from build123d import *

# Parameters (mm, degrees)
EXTRUDE_1_DEPTH     = 1.2
SKETCH_2_R          = 1.375
CUT_EXTRUDE_1_DEPTH = 1.2
SKETCH_3_W          = 6
SKETCH_3_H          = 13
EXTRUDE_2_DEPTH     = 5
SKETCH_4_W          = 6
SKETCH_4_H          = 5
EXTRUDE_3_DEPTH     = 0.3
SKETCH_5_W          = 8
SKETCH_5_H          = 7
EXTRUDE_4_DEPTH     = 5.5
SKETCH_6_W          = 12
SKETCH_6_H          = 8.2
EXTRUDE_5_DEPTH     = 5.1
SKETCH_7_W          = 12
SKETCH_7_H          = 8.2
EXTRUDE_6_DEPTH     = 5.1
SKETCH_8_W          = 5.7
SKETCH_8_H          = 7.6
EXTRUDE_7_DEPTH     = 2.4
SKETCH_9_W          = 7.6
SKETCH_9_H          = 2.4
EXTRUDE_8_DEPTH     = 0.7
SKETCH_10_W         = 12
SKETCH_10_H         = 5.1
SKETCH_10_W_2       = 8
SKETCH_10_H_2       = 5.5
CUT_EXTRUDE_2_DEPTH = 0.5
SKETCH_11_W         = 51.4
SKETCH_11_H         = 5.1
EXTRUDE_9_DEPTH     = 8.5
SKETCH_12_W         = 6.2
SKETCH_12_H         = 6.2
EXTRUDE_10_DEPTH    = 3.5
SKETCH_13_R         = 1.75
EXTRUDE_11_DEPTH    = 1.5
SKETCH_14_W         = 2
SKETCH_14_H         = 2
EXTRUDE_12_DEPTH    = 1
SKETCH_15_R         = 2.75
SKETCH_15_R_2       = 1.55
EXTRUDE_13_DEPTH    = 2


with BuildPart() as part:
    # 草图1 → 凸台-拉伸1 (new body)
    with BuildSketch(Plane(origin=(0, 0, 0), x_dir=(1, 0, 0), z_dir=(0, 1, 0))):
        with BuildLine():
            Line((-29.5, 15), (29.5, 15))
            ThreePointArc((29.5, 15), (31.621320344, 14.121320344), (32.5, 12))
            Line((32.5, 12), (32.5, -12))
            ThreePointArc((32.5, -12), (31.621320344, -14.121320344), (29.5, -15))
            Line((29.5, -15), (-29.5, -15))
            ThreePointArc((-29.5, -15), (-31.621320344, -14.121320344), (-32.5, -12))
            Line((-32.5, -12), (-32.5, 12))
            ThreePointArc((-32.5, 12), (-31.621320344, 14.121320344), (-29.5, 15))
        make_face()
    extrude(amount=EXTRUDE_1_DEPTH)

    # 草图2 → 切除-拉伸1 (cut)
    with BuildSketch(Plane(origin=(0, 1.2, 0), x_dir=(1, 0, 0), z_dir=(0, 1, 0))):
        with Locations(Location((29, -11.5, 0), (0, 0, 270))):
            Circle(SKETCH_2_R)
        with Locations(Location((29, 11.5, 0), (0, 0, 270))):
            Circle(SKETCH_2_R)
        with Locations(Location((-29, -11.5, 0), (0, 0, 270))):
            Circle(SKETCH_2_R)
        with Locations(Location((-29, 11.5, 0), (0, 0, 270))):
            Circle(SKETCH_2_R)
    extrude(amount=-CUT_EXTRUDE_1_DEPTH, mode=Mode.SUBTRACT)

    # 草图3 → 凸台-拉伸2 (add)
    with BuildSketch(Plane(origin=(0, 1.2, 0), x_dir=(1, 0, 0), z_dir=(0, 1, 0))):
        with Locations((22.3, -8.5)):
            Rectangle(SKETCH_3_W, SKETCH_3_H)
    extrude(amount=EXTRUDE_2_DEPTH)

    # 草图4 → 凸台-拉伸3 (add)
    with BuildSketch(Plane.XY.offset(15)):
        with Locations((22.3, 3.7)):
            Rectangle(SKETCH_4_W, SKETCH_4_H)
    extrude(amount=EXTRUDE_3_DEPTH)

    # 草图5 → 凸台-拉伸4 (add)
    with BuildSketch(Plane(origin=(0, 1.2, 0), x_dir=(1, 0, 0), z_dir=(0, 1, 0))):
        with Locations((5.6, -11.5)):
            Rectangle(SKETCH_5_W, SKETCH_5_H)
    extrude(amount=EXTRUDE_4_DEPTH)

    # 草图6 → 凸台-拉伸5 (add)
    with BuildSketch(Plane(origin=(0, 1.2, 0), x_dir=(1, 0, 0), z_dir=(0, 1, 0))):
        with Locations((-5.9, -10.9)):
            Rectangle(SKETCH_6_W, SKETCH_6_H)
    extrude(amount=EXTRUDE_5_DEPTH)

    # 草图7 → 凸台-拉伸6 (add)
    with BuildSketch(Plane(origin=(0, 1.2, 0), x_dir=(1, 0, 0), z_dir=(0, 1, 0))):
        with Locations((-19.45, -10.9)):
            Rectangle(SKETCH_7_W, SKETCH_7_H)
    extrude(amount=EXTRUDE_6_DEPTH)

    # 草图8 → 凸台-拉伸7 (add)
    with BuildSketch(Plane(origin=(0, 1.2, 0), x_dir=(1, 0, 0), z_dir=(0, 1, 0))):
        with Locations((-29.65, -1.5)):
            Rectangle(SKETCH_8_W, SKETCH_8_H)
    extrude(amount=EXTRUDE_7_DEPTH)

    # 草图9 → 凸台-拉伸8 (add)
    with BuildSketch(Plane.ZY.offset(32.5)):
        with Locations((1.5, 2.4)):
            Rectangle(SKETCH_9_W, SKETCH_9_H)
    extrude(amount=EXTRUDE_8_DEPTH)

    # 草图10 → 切除-拉伸2 (cut)
    with BuildSketch(Plane.XY.offset(15)):
        with Locations((-19.45, 3.75)):
            Rectangle(SKETCH_10_W, SKETCH_10_H)
        with Locations((-5.9, 3.75)):
            Rectangle(SKETCH_10_W, SKETCH_10_H)
        with Locations((5.6, 3.95)):
            Rectangle(SKETCH_10_W_2, SKETCH_10_H_2)
    extrude(amount=-CUT_EXTRUDE_2_DEPTH, mode=Mode.SUBTRACT)

    # 草图11 → 凸台-拉伸9 (add)
    with BuildSketch(Plane.XZ):
        with Locations((-0.05, -11.55)):
            Rectangle(SKETCH_11_W, SKETCH_11_H)
    extrude(amount=EXTRUDE_9_DEPTH)

    # 草图12 → 凸台-拉伸10 (add)
    with BuildSketch(Plane(origin=(0, 1.2, 0), x_dir=(1, 0, 0), z_dir=(0, 1, 0))):
        with Locations((-16.2, 2.6)):
            Rectangle(SKETCH_12_W, SKETCH_12_H)
    extrude(amount=EXTRUDE_10_DEPTH)

    # 草图13 → 凸台-拉伸11 (add)
    with BuildSketch(Plane(origin=(0, 4.7, 0), x_dir=(1, 0, 0), z_dir=(0, 1, 0))):
        with Locations(Location((-16.2, 2.6, 0), (0, 0, 270))):
            Circle(SKETCH_13_R)
    extrude(amount=EXTRUDE_11_DEPTH)

    # 草图14 → 凸台-拉伸12 (add)
    with BuildSketch(Plane(origin=(0, 1.2, 0), x_dir=(1, 0, 0), z_dir=(0, 1, 0))):
        with Locations((3.2, 3.22)):
            Rectangle(SKETCH_14_W, SKETCH_14_H)
        with Locations((0, 3.22)):
            Rectangle(SKETCH_14_W, SKETCH_14_H)
        with Locations((-3.2, 3.22)):
            Rectangle(SKETCH_14_W, SKETCH_14_H)
    extrude(amount=EXTRUDE_12_DEPTH)

    # 草图15 → 凸台-拉伸13 (add)
    with BuildSketch(Plane.XY.offset(15.3)):
        with Locations(Location((22.3, 3.7, 0), (0, 0, 114.619977329))):
            Circle(SKETCH_15_R)
        with Locations((22.3, 3.7)):
            Circle(SKETCH_15_R_2, mode=Mode.SUBTRACT)
    extrude(amount=EXTRUDE_13_DEPTH)


solid = part.part
The listing builds one solid part. Answer for the finished solid, in the listing's coordinates (mm). A direction names the side the tool comes from. Round coordinates to 2 decimals unless told otherwise and drop trailing zeros. Order: outer loops, then holes, each group sorted by start corner. A loop starts at its lowest first (then second) coordinate and runs counter-clockwise, first axis right, second up. Notation, with made-up numbers: (-2.75, 51.25) -> (21.25, 51.25) arc R17 ccw to (21.25, 60.25) -> close; hole circle Ø3 at (-11.75, -7). An arc over 180 degrees is marked (long way). Put each result on its own line as item: value.
Q1. Each of these flat-tipped pins is pushed along its axis until it touches: P1, Ø9, axis at x = 4.5, z = -1.5, coming from the +Y side; P2, Ø12, axis at x = -16.5, z = 7.5, coming from the -Y side; P3, Ø1.9, axis at x = -15, z = -2, coming from the +Y side; P4, Ø1, axis at y = -1, z = -7.5, coming from the -X side. Where does it stop, or does it pass through?
Results list:
P1: y = 2.2
P2: y = 0
P3: y = 6.2
P4: through
Q2. Which of the six approach directions +Z, -Z, +X, -X, +Y, -Y give full straight-line access (tool end or side, diameter ignored) to faces 1 (the flat face through (-19.3, 3, -3)), 2 (the flat face through (-16, 6.2, -3)), 3 (the flat face through (19.3, 4, 9))?
Results list:
face 1: -Z, +Y
face 2: -Z, +X, -X, +Y
face 3: +Z, -Z, +Y
Q3. Section D-D, the plane y = -1 is taken. Write down the section's boundary in (x, z), and give its area (3 significant figures).
Results list:
outline: (-25.75, -14.1) -> (25.65, -14.1) -> (25.65, -9) -> (-25.75, -9) -> close
area: 262 mm^2
Q4. Consider line 1 along X through (y, z) = (0.7, -11.5) (3 decimals); line 2 along X through (y, z) = (4.5, 12.5); line 3 along X through (y, z) = (1.25, -1). Determine where each line is inside the solid, lowest interval first.
Results list:
line 1: -32.5 to -30.375, -27.625 to 27.625, 30.375 to 32.5
line 2: -25.45 to -13.45, -11.9 to 0.1, 1.6 to 9.6, 19.3 to 25.3
line 3: -33.2 to -26.8, -19.3 to -13.1
Q5. Determine the mould class of faces 4 (the flat face through (-6, 4, 14.5)), 5 (the flat face through (-16, 3, -5.7)), 6 (the flat face through (-25.75, -4, -12)), 7 (the flat face through (-20, 4, 6.8)) for opening direction Z: pulls with the +Z half, pulls with the -Z half, needs draft (parallel to the pull), parting line crosses it, or undercut.
Results list:
face 4: pulls with the +Z half
face 5: pulls with the -Z half
face 6: needs draft
face 7: undercut
Q6. Section C-C, the plane y = 3 is taken. Count the separate pieces of the cut face and the enclosed holes in it, and give its area (3 significant figures).
Results list:
separate pieces: 6
enclosed holes: 0
area: 409 mm^2
Q7. Section A-A, the plane z = -11 is taken. Write down the section's boundary in (x, y).
Results list:
outline: (-32.5, 0) -> (-30.28, 0) -> (-30.28, 1.2) -> (-32.5, 1.2) -> close; (-27.72, 0) -> (-25.75, 0) -> (-25.75, -8.5) -> (25.65, -8.5) -> (25.65, 0) -> (27.72, 0) -> (27.72, 1.2) -> (-27.72, 1.2) -> close; (30.28, 0) -> (32.5, 0) -> (32.5, 1.2) -> (30.28, 1.2) -> close
Q8. Section B-B, the plane x = -5 is taken. Write down the section's boundary in (y, z).
Results list:
outline: (-8.5, -14.1) -> (0, -14.1) -> (0, -15) -> (1.2, -15) -> (1.2, 6.8) -> (6.3, 6.8) -> (6.3, 14.5) -> (1.2, 14.5) -> (1.2, 15) -> (0, 15) -> (0, -9) -> (-8.5, -9) -> close
